```python
from build123d import *

# Parameters (mm, degrees)
SKETCH10_R              = 5
BOSS_EXTRUDE1_DEPTH     = 100
SKETCH11_W              = 10
SKETCH11_H              = 15
CUT_EXTRUDE1_DEPTH      = 100
SKETCH12_R              = 1.6
CUT_EXTRUDE2_DEPTH      = 101.369318021
MIRROR8_COPY_1_SKETCH_W = 10
MIRROR8_COPY_1_SKETCH_H = 15
MIRROR8_COPY_1_DEPTH    = 100
MIRROR8_COPY_2_SKETCH_W = 10
MIRROR8_COPY_2_SKETCH_H = 15
MIRROR8_COPY_2_DEPTH    = 100
FILLET1_R               = 4
FILLET2_R               = 4


with BuildPart() as part:
    # Sketch10 → Boss-Extrude1 (new body)
    with BuildSketch(Plane(origin=(0, 0, 0), x_dir=(1, 0, 0), z_dir=(0, 1, 0))):
        with Locations(Location((0, 0, 0), (0, 0, 270))):
            Circle(SKETCH10_R)
    extrude(amount=BOSS_EXTRUDE1_DEPTH)

    # Sketch11 → Cut-Extrude1 (cut)
    with BuildSketch(Plane(origin=(2, 0, 0), x_dir=(0, 0, -1), z_dir=(1, 0, 0))):
        with Locations((0, 7.5)):
            Rectangle(SKETCH11_W, SKETCH11_H)
    cut_extrude1 = extrude(amount=CUT_EXTRUDE1_DEPTH, mode=Mode.SUBTRACT)

    # Mirror1: Cut-Extrude1 across plane
    add(cut_extrude1.mirror(Plane(origin=(0, 0, 0), x_dir=(0, 0, 1), z_dir=(1, 0, 0))), mode=Mode.SUBTRACT)

    # Sketch12 → Cut-Extrude2 (cut, through all)
    with BuildSketch(Plane.ZY.offset(2)):
        with Locations((0, 7)):
            Circle(SKETCH12_R)
    cut_extrude2 = extrude(amount=-CUT_EXTRUDE2_DEPTH, mode=Mode.SUBTRACT)

    # Mirror7: Cut-Extrude1 across plane
    add(cut_extrude1.mirror(Plane(origin=(0, 50, 0), x_dir=(0, 0, 1), z_dir=(0, -1, 0))), mode=Mode.SUBTRACT)

    # Mirror8 copy 1 sketch → Mirror8 copy 1 (cut)
    with BuildSketch(Plane(origin=(-2, 100, 0), x_dir=(0, 0, -1), z_dir=(-1, 0, 0))):
        with Locations((0, 7.5)):
            Rectangle(MIRROR8_COPY_1_SKETCH_W, MIRROR8_COPY_1_SKETCH_H)
    extrude(amount=MIRROR8_COPY_1_DEPTH, mode=Mode.SUBTRACT)

    # Mirror8 copy 2 sketch → Mirror8 copy 2 (cut)
    with BuildSketch(Plane(origin=(2, 100, 0), x_dir=(0, 0, -1), z_dir=(1, 0, 0))):
        with Locations((0, -7.5)):
            Rectangle(MIRROR8_COPY_2_SKETCH_W, MIRROR8_COPY_2_SKETCH_H)
    extrude(amount=MIRROR8_COPY_2_DEPTH, mode=Mode.SUBTRACT)

    # Mirror9: Cut-Extrude2 across plane
    add(cut_extrude2.mirror(Plane(origin=(0, 50, 0), x_dir=(0, 0, 1), z_dir=(0, -1, 0))), mode=Mode.SUBTRACT)

    # Fillet1
    # the kernel refuses this fillet: 4 mm, written as the material it takes off along each edge
    with BuildSketch(Plane(origin=(0, 15, 0), x_dir=(0.9999950652018581, 0, 0.003141587485879613), z_dir=(0.003141587485879613, 0, -0.9999950652018581))) as fillet1_piece_1_section:
        with BuildLine():
            CenterArc((5 - FILLET1_R, -FILLET1_R), FILLET1_R, 0, 90)
            Line((5 - FILLET1_R, 0), (5, 0))
            Line((5, 0), (5, -FILLET1_R))
        make_face()
    fillet1_piece_1 = revolve(axis=Axis((0, 15, 0), (0, -1, 0)), revolution_arc=359.64, mode=Mode.PRIVATE)
    fillet1_piece_1 = split(fillet1_piece_1, bisect_by=Plane(origin=(2, 16.020930517, 2.132715254), z_dir=(1, 0, 0)), keep=Keep.TOP, mode=Mode.PRIVATE)
    add(fillet1_piece_1, mode=Mode.SUBTRACT)
    with BuildSketch(Plane(origin=(0, 15, 0), x_dir=(0.9999950652018581, 0, 0.003141587485879613), z_dir=(0.003141587485879613, 0, -0.9999950652018581))) as fillet1_piece_2_section:
        with BuildLine():
            CenterArc((5 - FILLET1_R, -FILLET1_R), FILLET1_R, 0, 90)
            Line((5 - FILLET1_R, 0), (5, 0))
            Line((5, 0), (5, -FILLET1_R))
        make_face()
    fillet1_piece_2 = revolve(axis=Axis((0, 15, 0), (0, -1, 0)), revolution_arc=359.64, mode=Mode.PRIVATE)
    fillet1_piece_2 = split(fillet1_piece_2, bisect_by=Plane(origin=(-2, 16.531416738, 0), z_dir=(-1, 0, 0)), keep=Keep.TOP, mode=Mode.PRIVATE)
    add(fillet1_piece_2, mode=Mode.SUBTRACT)
    with BuildSketch(Plane(origin=(0, 15, 0), x_dir=(-0.9999950652018581, 0, -0.0031415874858794907), z_dir=(-0.0031415874858794907, 0, 0.9999950652018581))) as fillet1_piece_3_section:
        with BuildLine():
            CenterArc((5 - FILLET1_R, -FILLET1_R), FILLET1_R, 0, 90)
            Line((5 - FILLET1_R, 0), (5, 0))
            Line((5, 0), (5, -FILLET1_R))
        make_face()
    fillet1_piece_3 = revolve(axis=Axis((0, 15, 0), (0, -1, 0)), revolution_arc=359.64, mode=Mode.PRIVATE)
    fillet1_piece_3 = split(fillet1_piece_3, bisect_by=Plane(origin=(-2, 16.020930615, -2.132715254), z_dir=(-1, 0, 0)), keep=Keep.TOP, mode=Mode.PRIVATE)
    add(fillet1_piece_3, mode=Mode.SUBTRACT)
    with BuildSketch(Plane(origin=(0, 15, 0), x_dir=(-0.9999950652018581, 0, -0.0031415874858794907), z_dir=(-0.0031415874858794907, 0, 0.9999950652018581))) as fillet1_piece_4_section:
        with BuildLine():
            CenterArc((5 - FILLET1_R, -FILLET1_R), FILLET1_R, 0, 90)
            Line((5 - FILLET1_R, 0), (5, 0))
            Line((5, 0), (5, -FILLET1_R))
        make_face()
    fillet1_piece_4 = revolve(axis=Axis((0, 15, 0), (0, -1, 0)), revolution_arc=359.64, mode=Mode.PRIVATE)
    fillet1_piece_4 = split(fillet1_piece_4, bisect_by=Plane(origin=(2, 16.531416738, 0), z_dir=(1, 0, 0)), keep=Keep.TOP, mode=Mode.PRIVATE)
    add(fillet1_piece_4, mode=Mode.SUBTRACT)
    with BuildSketch(Plane(origin=(0, 85, 0), x_dir=(-0.9999950652018581, 0, -0.0031415874858794907), z_dir=(-0.0031415874858794907, 0, 0.9999950652018581))) as fillet1_piece_5_section:
        with BuildLine():
            CenterArc((5 - FILLET1_R, FILLET1_R), FILLET1_R, 270, 90)
            Line((5 - FILLET1_R, 0), (5, 0))
            Line((5, 0), (5, FILLET1_R))
        make_face()
    fillet1_piece_5 = revolve(axis=Axis((0, 85, 0), (0, -1, 0)), revolution_arc=359.64, mode=Mode.PRIVATE)
    fillet1_piece_5 = split(fillet1_piece_5, bisect_by=Plane(origin=(-2, 83.979069385, -2.132715254), z_dir=(-1, 0, 0)), keep=Keep.TOP, mode=Mode.PRIVATE)
    add(fillet1_piece_5, mode=Mode.SUBTRACT)
    with BuildSketch(Plane(origin=(0, 85, 0), x_dir=(-0.9999950652018581, 0, -0.0031415874858794907), z_dir=(-0.0031415874858794907, 0, 0.9999950652018581))) as fillet1_piece_6_section:
        with BuildLine():
            CenterArc((5 - FILLET1_R, FILLET1_R), FILLET1_R, 270, 90)
            Line((5 - FILLET1_R, 0), (5, 0))
            Line((5, 0), (5, FILLET1_R))
        make_face()
    fillet1_piece_6 = revolve(axis=Axis((0, 85, 0), (0, -1, 0)), revolution_arc=359.64, mode=Mode.PRIVATE)
    fillet1_piece_6 = split(fillet1_piece_6, bisect_by=Plane(origin=(2, 83.468583262, 0), z_dir=(1, 0, 0)), keep=Keep.TOP, mode=Mode.PRIVATE)
    add(fillet1_piece_6, mode=Mode.SUBTRACT)
    with BuildSketch(Plane(origin=(0, 85, 0), x_dir=(0.9999950652018581, 0, 0.003141587485879613), z_dir=(0.003141587485879613, 0, -0.9999950652018581))) as fillet1_piece_7_section:
        with BuildLine():
            CenterArc((5 - FILLET1_R, FILLET1_R), FILLET1_R, 270, 90)
            Line((5 - FILLET1_R, 0), (5, 0))
            Line((5, 0), (5, FILLET1_R))
        make_face()
    fillet1_piece_7 = revolve(axis=Axis((0, 85, 0), (0, -1, 0)), revolution_arc=359.64, mode=Mode.PRIVATE)
    fillet1_piece_7 = split(fillet1_piece_7, bisect_by=Plane(origin=(2, 83.979069483, 2.132715254), z_dir=(1, 0, 0)), keep=Keep.TOP, mode=Mode.PRIVATE)
    add(fillet1_piece_7, mode=Mode.SUBTRACT)
    with BuildSketch(Plane(origin=(0, 85, 0), x_dir=(0.9999950652018581, 0, 0.003141587485879613), z_dir=(0.003141587485879613, 0, -0.9999950652018581))) as fillet1_piece_8_section:
        with BuildLine():
            CenterArc((5 - FILLET1_R, FILLET1_R), FILLET1_R, 270, 90)
            Line((5 - FILLET1_R, 0), (5, 0))
            Line((5, 0), (5, FILLET1_R))
        make_face()
    fillet1_piece_8 = revolve(axis=Axis((0, 85, 0), (0, -1, 0)), revolution_arc=359.64, mode=Mode.PRIVATE)
    fillet1_piece_8 = split(fillet1_piece_8, bisect_by=Plane(origin=(-2, 83.468583262, 0), z_dir=(-1, 0, 0)), keep=Keep.TOP, mode=Mode.PRIVATE)
    add(fillet1_piece_8, mode=Mode.SUBTRACT)

    # Fillet2
    # the kernel refuses this fillet: 4 mm, written as the material it takes off along each edge
    with BuildSketch(Plane(origin=(0, 0, 0), x_dir=(-0.6668850456417628, 0, -0.7451606108077533), z_dir=(0.7451606108077533, 0, -0.6668850456417628))) as fillet2_piece_1:
        with BuildLine():
            CenterArc((5 - FILLET2_R, FILLET2_R), FILLET2_R, 270, 90)
            Line((5 - FILLET2_R, 0), (5, 0))
            Line((5, 0), (5, FILLET2_R))
        make_face()
    revolve(axis=Axis((0, 0, 0), (0, 1, 0)), revolution_arc=138.172896035, mode=Mode.SUBTRACT)
    with BuildSketch(Plane(origin=(0, 0, 0), x_dir=(0.6667617921571638, 0, 0.7452708987471381), z_dir=(-0.7452708987471381, 0, 0.6667617921571638))) as fillet2_piece_2:
        with BuildLine():
            CenterArc((5 - FILLET2_R, FILLET2_R), FILLET2_R, 270, 90)
            Line((5 - FILLET2_R, 0), (5, 0))
            Line((5, 0), (5, FILLET2_R))
        make_face()
    revolve(axis=Axis((0, 0, 0), (0, 1, 0)), revolution_arc=276.364744713, mode=Mode.SUBTRACT)
    with BuildSketch(Plane(origin=(0, 100, 0), x_dir=(-0.6668850456417623, 0, -0.7451606108077536), z_dir=(0.7451606108077536, 0, -0.6668850456417623))) as fillet2_piece_3:
        with BuildLine():
            CenterArc((5 - FILLET2_R, -FILLET2_R), FILLET2_R, 0, 90)
            Line((5 - FILLET2_R, 0), (5, 0))
            Line((5, 0), (5, -FILLET2_R))
        make_face()
    revolve(axis=Axis((0, 100, 0), (0, 1, 0)), revolution_arc=138.172896035, mode=Mode.SUBTRACT)
    with BuildSketch(Plane(origin=(0, 100, 0), x_dir=(0.6667617921571635, 0, 0.7452708987471385), z_dir=(-0.7452708987471385, 0, 0.6667617921571635))) as fillet2_piece_4:
        with BuildLine():
            CenterArc((5 - FILLET2_R, -FILLET2_R), FILLET2_R, 0, 90)
            Line((5 - FILLET2_R, 0), (5, 0))
            Line((5, 0), (5, -FILLET2_R))
        make_face()
    revolve(axis=Axis((0, 100, 0), (0, 1, 0)), revolution_arc=276.364744713, mode=Mode.SUBTRACT)
    with BuildSketch(Plane(origin=(0, 100, 0), x_dir=(0, 0, 1), z_dir=(-1, 0, 0))) as fillet2_piece_5:
        with BuildLine():
            CenterArc((5 - FILLET2_R, -FILLET2_R), FILLET2_R, 0, 90)
            Line((5 - FILLET2_R, 0), (5, 0))
            Line((5, 0), (5, -FILLET2_R))
        make_face()
    revolve(axis=Axis((0, 100, 0), (0, 1, 0)), revolution_arc=138.172896035, mode=Mode.SUBTRACT)
    with BuildSketch(Plane(origin=(0, 0, 0), x_dir=(0, 0, 1), z_dir=(-1, 0, 0))) as fillet2_piece_6:
        with BuildLine():
            CenterArc((5 - FILLET2_R, FILLET2_R), FILLET2_R, 270, 90)
            Line((5 - FILLET2_R, 0), (5, 0))
            Line((5, 0), (5, FILLET2_R))
        make_face()
    revolve(axis=Axis((0, 0, 0), (0, 1, 0)), revolution_arc=138.172896035, mode=Mode.SUBTRACT)


solid = part.part
```
Geometry: final body of the model. Coordinates: model frame, mm. Round coordinates to 2 decimals unless told otherwise and drop trailing zeros. Order: outer loops, then holes, each group sorted by start corner. A loop starts at its lowest first (then second) coordinate and runs counter-clockwise, first axis right, second up. Notation, with made-up numbers: (-11.5, 17) - (41.5, 17) arc R16 cw to (41.5, 38) - close; hole circle Ø4 at (37, 75.5). An arc over 180 degrees is marked (long way). Write item = value, one per line. Start each with the question number.
Q1. Cut plane A-A on y = 7. Return the cut outline in (x, z), and give its area (3 significant figures).
Q2. Pin query (flat end, axial travel): pin 1 (5 mm diameter, centred on y = 93, z = 0, fed in from +X); pin 2 (2.5 mm diameter, centred on y = 14, z = 2, fed in from -X); pin 3 (1 mm diameter, centred on x = -4, y = 17.5, fed in from +Z). Return the tip coordinate at first contact, or that it passes through.
Q3. Cut plane B-B on y = 20.5. Return the cut outline in (x, z), and give its area (3 significant figures).
Q4. Pull-direction query (Y, two-part tool) for faces 1 (the cylindrical face through (1.5, 49.36, 4.77)), 2 (the flat face through (0, 100, 0)), 3 (the cylindrical face through (-0.03, 5.44, -0.35)); classes: +Y half, -Y half, draft (parallel to the pull), parting line (faces both ways), or undercut.
Q5. Ray query, line 1 (Y direction, x = 0, z = 0); line 2 (X direction, y = 75.5, z = 2); line 3 (Z direction, x = 0.45, y = 93). Return the intervals inside material, ascending. Write a range as from..to.
Outcome:
q1.outline = (-2, -4.58) arc R5 ccw to (2, -4.58) - (2, -1.6) - (-2, -1.6) - close; (-2, 1.6) - (2, 1.6) - (2, 4.58) arc R5 ccw to (-2, 4.58) - close
q1.area = 26.1 mm^2
q2.pin_1 = 2
q2.pin_2 = -2
q2.pin_3 = 3.21
q3.outline = circle Ø10 at (0, 0)
q3.area = 78.5 mm^2
q4.face_1 = draft
q4.face_2 = +Y half
q4.face_3 = undercut
q5.line_1 = 0..5.4, 8.6..91.4, 94.6..100
q5.line_2 = -4.58..4.58
q5.line_3 = -4.98..-1.6, 1.6..4.98
